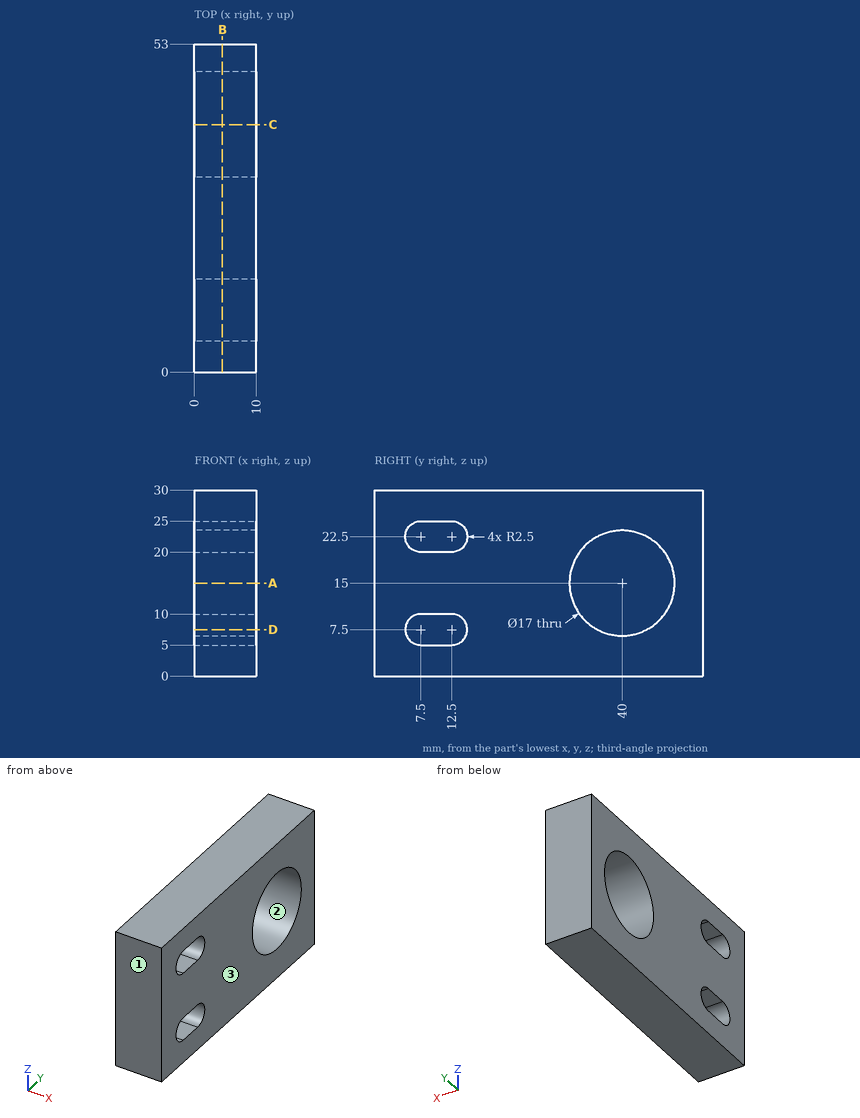
For this review, use the dimensioned drawing (mm, ordinates from the lowest corner) and the shaded views. Round coordinates to 2 decimals unless told otherwise and drop trailing zeros. Order: outer loops, then holes, each group sorted by start corner. A loop starts at its lowest first (then second) coordinate and runs counter-clockwise, first axis right, second up. Notation, with made-up numbers: M 61,40.5 L 110,40.5 A12 cw 110,52.5 Z; hole C 40,-37.75 d11. An arc over 180 degrees is marked long. Use a Markdown table: item, result.
1) Consider section A-A (z = 15). Write out the cut boundary in (x, y), then the cut area to 3 significant figures.
Report:
| item | result |
|---|---|
| outline | M 0,0 L 10,0 L 10,31.5 L 0,31.5 Z; M 0,48.5 L 10,48.5 L 10,53 L 0,53 Z |
| area | 360 mm^2 |
2) Consider section C-C (y = 40). Write out the cut boundary in (x, z).
Report:
| item | result |
|---|---|
| outline | M 0,0 L 10,0 L 10,6.5 L 0,6.5 Z; M 0,23.5 L 10,23.5 L 10,30 L 0,30 Z |
3) Wall thickness on line 1 along Z through (x, y) = (1.5, 12); line 2 along Y through (x, z) = (5.25, 15); line 3 along Z through (x, y) = (9.75, 6): over which ranges is each line inside the solid? List them lowest first. Write a range as [from, to].
Report:
| item | result |
|---|---|
| line 1 | [0, 5], [10, 20], [25, 30] |
| line 2 | [0, 31.5], [48.5, 53] |
| line 3 | [0, 5.5], [9.5, 20.5], [24.5, 30] |
4) Consider section B-B (x = 4.5). Write out the cut boundary in (y, z), then the cut area to 3 significant figures.
Report:
| item | result |
|---|---|
| outline | M 0,0 L 53,0 L 53,30 L 0,30 Z; hole M 7.5,5 L 12.5,5 A2.5 ccw 12.5,10 L 7.5,10 A2.5 ccw Z; hole M 7.5,20 L 12.5,20 A2.5 ccw 12.5,25 L 7.5,25 A2.5 ccw Z; hole C 40,15 d17 |
| area | 1,270 mm^2 |
5) Draft analysis for pull direction Y (two halves, no side actions). For the marked faces 1, 2 and 3, state which applies: released by +Y, released by -Y, zero draft, split by the parting line, or undercut.
Report:
| item | result |
|---|---|
| face 1 | released by -Y |
| face 2 | undercut |
| face 3 | zero draft |
6) Consider section D-D (z = 7.5). Write out the cut boundary in (x, y), then the cut area to 3 significant figures.
Report:
| item | result |
|---|---|
| outline | M 0,0 L 10,0 L 10,5 L 0,5 Z; M 0,15 L 10,15 L 10,36 L 0,36 Z; M 0,44 L 10,44 L 10,53 L 0,53 Z |
| area | 350 mm^2 |
